from build123d import *

# Parameters (mm, degrees)
SKETCH1_R           = 1.5
BOSS_EXTRUDE1_DEPTH = 3
SKETCH2_R           = 25
SKETCH2_R_2         = 8.35
BOSS_EXTRUDE2_DEPTH = 3


with BuildPart() as part:
    # Sketch1 → Boss-Extrude1 (new body)
    with BuildSketch(Plane(origin=(0, 0, 0), x_dir=(1, 0, 0), z_dir=(0, 1, 0))):
        with BuildLine():
            Line((50, 0), (50, 55.901699437))
            ThreePointArc((50, 55.901699437), (0, 75), (-50, 55.901699437))
            Line((-50, 55.901699437), (-50, 0))
            Line((-50, 0), (-50, -55.901699437))
            ThreePointArc((-50, -55.901699437), (0, -75), (50, -55.901699437))
            Line((50, -55.901699437), (50, 0))
        make_face()
        with Locations(Location((-40, -44.9, 0), (0, 0, 270))):
            Circle(SKETCH1_R, mode=Mode.SUBTRACT)
        with Locations(Location((-29.5, -40.4, 0), (0, 0, 270))):
            Circle(SKETCH1_R, mode=Mode.SUBTRACT)
        with Locations(Location((29.5, -40.4, 0), (0, 0, 270))):
            Circle(SKETCH1_R, mode=Mode.SUBTRACT)
        with Locations(Location((-29.5, 40.4, 0), (0, 0, 270))):
            Circle(SKETCH1_R, mode=Mode.SUBTRACT)
        with Locations(Location((29.5, 40.4, 0), (0, 0, 270))):
            Circle(SKETCH1_R, mode=Mode.SUBTRACT)
        with Locations(Location((40, 44.9, 0), (0, 0, 270))):
            Circle(SKETCH1_R, mode=Mode.SUBTRACT)
        with Locations(Location((-40, 44.9, 0), (0, 0, 270))):
            Circle(SKETCH1_R, mode=Mode.SUBTRACT)
        with Locations(Location((40, -44.9, 0), (0, 0, 270))):
            Circle(SKETCH1_R, mode=Mode.SUBTRACT)
    extrude(amount=BOSS_EXTRUDE1_DEPTH)

    # Sketch2 → Boss-Extrude2 (add)
    with BuildSketch(Plane(origin=(0, 3, 0), x_dir=(1, 0, 0), z_dir=(0, 1, 0))):
        with Locations(Location((0, 0, 0), (0, 0, 270))):
            Circle(SKETCH2_R)
        with Locations(Location((0, 0, 0), (0, 0, 270))):
            Circle(SKETCH2_R_2, mode=Mode.SUBTRACT)
    extrude(amount=BOSS_EXTRUDE2_DEPTH)


solid = part.part
Geometry: final body of the model. Coordinates: model frame, mm. A direction names the side the tool comes from. Give positions to 0.01 mm unless a question says otherwise; leave off trailing zeros. Write each loop counter-clockwise with the first axis right and the second up, starting at its lowest first coordinate (ties: lowest second). Pieces come first, ordered by that corner, then holes. Notation, with made-up numbers: M 7.25,-30.75 L 52.25,-30.75 A28 cw 52.25,-11.75 Z; hole C 15.5,72.5 d1. An arc over 180 degrees is marked long. Answer in a Markdown table with one row per item. Add a question column.
(1) Section A-A on z = -44.9. Return loops of the section in (x, y), and give its area (3 significant figures).
(2) Ray query, line 1 (X direction, y = 1.4, z = -44.9); line 2 (X direction, y = 0.85, z = 40.4); line 3 (Y direction, x = -0.5, z = 30). Return the intervals inside material, ascending.
(3) Section C-C on z = 0. Return loops of the section in (x, y), and give its area (3 significant figures).
(4) Reachability of faces 1 (the flat face through (-23, 3, 16)), 2 (the cylindrical face through (-28.49, 1.48, -41.51)) from +Z, -Z, +X, -X, +Y, -Y: full face, straight path, thin tool, end or side. Return the list, or none.
(5) First-contact query: pin 1 (6 mm diameter, centred on x = 4, z = 52, fed in from +Y); pin 2 (2.5 mm diameter, centred on x = -40, z = 44.9, fed in from +Y); pin 3 (1 mm diameter, centred on x = 18.5, y = 3, fed in from +Z). Flat tips, straight axial feed; report the tip coordinate or a pass-through.
(6) Section D-D on y = 4.6. Return loops of the section in (x, z).
(7) Section B-B on x = -40. Return loops of the section in (y, z), and give its area (3 significant figures).
(8) Mould query, pull axis Z, two halves, no side actions, for faces 3 (the flat face through (-50, 1, -1)), 4 (the cylindrical face through (-40.575, 1.479, 46.286)), 5 (the cylindrical face through (-0.766, 1.479, 74.996)). Classes: +Z half, -Z half, draft (parallel to the pull), parting line (faces both ways), or undercut.
Result set:
| question | item | result |
|---|---|---|
| 1 | outline | M -50,0 L -41.5,0 L -41.5,3 L -50,3 Z; M -38.5,0 L 38.5,0 L 38.5,3 L -38.5,3 Z; M 41.5,0 L 50,0 L 50,3 L 41.5,3 Z |
| 1 | area | 282 mm^2 |
| 2 | line 1 | x = -50 to -41.5, -38.5 to 38.5, 41.5 to 50 |
| 2 | line 2 | x = -50 to -31, -28 to 28, 31 to 50 |
| 2 | line 3 | y = 0 to 3 |
| 3 | outline | M -50,0 L 50,0 L 50,3 L 25,3 L 25,6 L 8.35,6 L 8.35,3 L -8.35,3 L -8.35,6 L -25,6 L -25,3 L -50,3 Z |
| 3 | area | 400 mm^2 |
| 4 | face 1 | +Y |
| 4 | face 2 | +Y, -Y |
| 5 | pin 1 | stops at y = 3 |
| 5 | pin 2 | passes through |
| 5 | pin 3 | stops at z = 72.81 |
| 6 | outline | C 0,0 d50; hole C 0,0 d16.7 |
| 7 | outline | M 0,-63.44 L 3,-63.44 L 3,-46.4 L 0,-46.4 Z; M 0,-43.4 L 3,-43.4 L 3,43.4 L 0,43.4 Z; M 0,46.4 L 3,46.4 L 3,63.44 L 0,63.44 Z |
| 7 | area | 363 mm^2 |
| 8 | face 3 | draft |
| 8 | face 4 | undercut |
| 8 | face 5 | +Z half |
